Check sheet for the modelled part. Datum: model origin and axes. Units: mm. A direction names the side the tool comes from. Round coordinates to 2 decimals unless told otherwise and drop trailing zeros. Order: outer loops, then holes, each group sorted by start corner. A loop starts at its lowest first (then second) coordinate and runs counter-clockwise, first axis right, second up.
```python
from build123d import *

# Parameters (mm, degrees)
F1_DEPTH  = 66
F2_R      = 1.5
F3_DEPTH  = 25
F4_R      = 1
F5_DEPTH  = 25
F6_R      = 5
F7_R      = 6.5
F8_W      = 11.5
F8_H      = 48
F9_DEPTH  = 100
F11_DEPTH = 66


# Not quite as in the source:
# - a feature names something its author has since deleted; it is built from what else it names


with BuildPart() as f1:
    # F0 (on Top) → F1 (new body)
    with BuildSketch(Plane.XY):
        with BuildLine():
            Line((54.5, 33), (54.5, -24.9880321095))
            Line((54.5, -24.9880321095), (53.5, -27.7355095289))
            Line((53.5, -27.7355095289), (53.5, -31))
            Line((53.5, -31), (55, -31))
            Line((55, -31), (55, -28))
            Line((55, -28), (56, -25.2525225805))
            Line((56, -25.2525225805), (56, 33))
            ThreePointArc((56, 33), (54.5355339059, 36.5355339059), (51, 38))
            Line((51, 38), (-42.5, 38))
            ThreePointArc((-42.5, 38), (-46.0355339059, 36.5355339059), (-47.5, 33))
            Line((-47.5, 33), (-47.5, 0))
            Line((-47.5, 0), (-46.000000001, 0))
            Line((-46.000000001, 0), (-46.000000001, 33))
            ThreePointArc((-46.000000001, 33), (-44.9748737349, 35.4748737349), (-42.5, 36.500000001))
            Line((-42.5, 36.5), (51, 36.5))
            ThreePointArc((51, 36.5), (53.4748737342, 35.4748737342), (54.5, 33))
        make_face()
    extrude(amount=F1_DEPTH)

    # F2 (on face) → F3 (cut)
    with BuildSketch(Plane(origin=(0, 38, 0), x_dir=(-1, 0, 0), z_dir=(0, 1, 0))):
        with Locations((-38.75, 58)):
            Circle(F2_R)
        with Locations((-38.75, 8)):
            Circle(F2_R)
    extrude(amount=-F3_DEPTH, mode=Mode.SUBTRACT)

    # F4 (on face) → F5 (cut)
    with BuildSketch(Plane.YZ.offset(56)):
        with BuildLine():
            Line((-17, 58), (-21, 58))
            ThreePointArc((-21, 58), (-23.1213203436, 57.1213203436), (-24, 55))
            Line((-24, 55), (-24, 11))
            ThreePointArc((-24, 11), (-23.1213203436, 8.8786796564), (-21, 8))
            Line((-21, 8), (-17, 8))
            ThreePointArc((-17, 8), (-14.8786796564, 8.8786796564), (-14, 11))
            Line((-14, 11), (-14, 55))
            ThreePointArc((-14, 55), (-14.8786796564, 57.1213203436), (-17, 58))
        make_face()
        with BuildLine():
            Line((24, 58), (-5, 58))
            ThreePointArc((-5, 58), (-7.1213203436, 57.1213203436), (-8, 55))
            Line((-8, 55), (-8, 11))
            ThreePointArc((-8, 11), (-7.1213203436, 8.8786796564), (-5, 8))
            Line((-5, 8), (24, 8))
            ThreePointArc((24, 8), (26.1213203436, 8.8786796564), (27, 11))
            Line((27, 11), (27, 55))
            ThreePointArc((27, 55), (26.1213203436, 57.1213203436), (24, 58))
        make_face()
        with Locations((-19, 61)):
            Circle(F4_R)
        with Locations((9.5, 61)):
            Circle(F4_R)
        with Locations((9.5, 5)):
            Circle(F4_R)
        with Locations((-19, 5)):
            Circle(F4_R)
    extrude(amount=-F5_DEPTH, mode=Mode.SUBTRACT)

    # F6
    f6_edges = [f1.edges().sort_by_distance(p)[0] for p in [
        (55, -28, 33),
        (54.5, -24.988032, 33),
    ]]
    fillet(f6_edges, radius=F6_R)

    # F7
    f7_edges = [f1.edges().sort_by_distance(p)[0] for p in [
        (56, -25.252523, 33),
        (53.5, -27.73551, 33),
    ]]
    fillet(f7_edges, radius=F7_R)

    # F8 (on Top) → F9 (cut)
    with BuildSketch(Plane.XY):
        with Locations((-43.75, 19)):
            Rectangle(F8_W, F8_H)
    extrude(amount=F9_DEPTH, mode=Mode.SUBTRACT)

    # F10 (on Top) → F11 (join)
    with BuildSketch(Plane.XY):
        with BuildLine():
            Line((-43.2462567555, 37), (-43.2462567555, 35.5))
            Line((-43.2462567555, 35.5), (-42.2462567555, 35.5))
            ThreePointArc((-42.2462567555, 35.5), (-41.3780158671, 35.5759612349), (-40.5361560388, 35.8015368961))
            Line((-40.5361560388, 35.8015368961), (-39.1970705016, 36.2889241728))
            ThreePointArc((-39.1970705016, 36.2889241728), (-38.6077686218, 36.4468271355), (-38, 36.5))
            Line((-38, 36.5), (-38, 38))
            ThreePointArc((-38, 38), (-38.8682408883, 37.9240387651), (-39.7101007166, 37.6984631039))
            Line((-39.7101007166, 37.6984631039), (-41.0491862538, 37.2110758272))
            ThreePointArc((-41.0491862538, 37.2110758272), (-41.6384881336, 37.0531728645), (-42.2462567555, 37))
            Line((-42.2462567555, 37), (-43.2462567555, 37))
        make_face()
    extrude(amount=F11_DEPTH)


solid = f1.part
```
Item 1: Go/stop test with flat-tipped pins: P1, Ø2.5, axis at y = -30, z = 42, coming from the -X side; P2, Ø0.5, axis at x = -42.5, z = 33.5, coming from the -Y side; P3, Ø8, axis at x = -13, z = 38.5, coming from the -Y side. Record where each tip stops, or that it passes through.
Answer:
P1: stops at x = 53.5
P2: stops at y = 35.5
P3: stops at y = 36.5
Item 2: Sectioned sample at A-A (y = 4.5). Record the cut outline in (x, z), and give its area (3 significant figures).
Answer:
outline: (54.5, 0) - (56, 0) - (56, 8) - (54.5, 8) - close; (54.5, 58) - (56, 58) - (56, 66) - (54.5, 66) - close
area: 24.0 mm2
Item 3: Sectioned sample at D-D (x = -31). Record the cut outline in (y, z).
Answer:
outline: (36.5, 0) - (38, 0) - (38, 66) - (36.5, 66) - close
Item 4: Scan lines: line 1 along Z through (x, y) = (55.45, 9.5); line 2 along Z through (x, y) = (38, 37); line 3 along X through (y, z) = (-14.5, 61.5). Record each from-to range of solid material in increasing order.
Answer:
line 1: z = 0 to 4, 6 to 8, 58 to 60, 62 to 66
line 2: z = 0 to 6.7, 9.3 to 56.7, 59.3 to 66
line 3: x = 54.5 to 56
Item 5: Sectioned sample at C-C (x = 38.75). Record the cut outline in (y, z).
Answer:
outline: (36.5, 0) - (38, 0) - (38, 6.5) - (36.5, 6.5) - close; (36.5, 9.5) - (38, 9.5) - (38, 56.5) - (36.5, 56.5) - close; (36.5, 59.5) - (38, 59.5) - (38, 66) - (36.5, 66) - close
Item 6: Access from +Z, -Z, +X, -X, +Y, -Y to the whole of each face (thin tool, end or side, straight path). Record for faces 5 (the cylindrical face through (53.6, -27.74, 33.46)), 6 (the flat face through (53.5, -30, 33)), 7 (the flat face through (55, -30, 33)), 8 (the cylindrical face through (53.45, 35.5, 32.54)).
Answer:
face 5: +Z, -Z, -X
face 6: +Z, -Z, -X, -Y
face 7: +Z, -Z, +X, -Y
face 8: +Z, -Z
Item 7: Release check for a two-part mould opening along Z. For faces 1 (the cylindrical face through (55.26, -23.1, 57.14)), 2 (the cylindrical face through (55.26, -14.9, 8.86)), 3 (the flat face through (10, 37, 66)), 4 (the flat face through (6, 36.5, 33)) record: released by +Z, released by -Z, zero draft, split by the parting line, or undercut.
Answer:
face 1: undercut
face 2: undercut
face 3: released by +Z
face 4: zero draft
Item 8: Sectioned sample at B-B (z = 52). State how many separate pieces and enclosed holes the cut face has, and give its area (3 significant figures).
Answer:
separate pieces: 3
enclosed holes: 0
area: 180 mm2
